from build123d import *

# Parameters (mm, degrees)
F1_DEPTH = 1.5875


with BuildPart() as f1:
    # F0 (on Front) → F1 (new body, symmetric)
    with BuildSketch(Plane.XZ):
        with BuildLine():
            Line((4.516544, 39.664961), (0, 39.664961))
            Line((0, 39.664961), (-4.516544, 39.664961))
            Line((-4.516544, 39.664961), (-8.198804, 45.188352))
            Line((-8.198804, 45.188352), (-8.198804, 39.664961))
            ThreePointArc((-8.198804, 39.664961), (-22.375505, 31.529893), (-36.552206, 39.664961))
            Line((-36.552206, 39.664961), (-63.432701, 39.664961))
            ThreePointArc((-63.432701, 39.664961), (-53.299794, 33.172534), (-54.963503, 21.253662))
            Line((-54.963503, 21.253662), (-38.393334, 21.253662))
            ThreePointArc((-38.393334, 21.253662), (-18.023802, 17.746605), (0, 7.629301))
            ThreePointArc((0, 7.629301), (18.023802, 17.746605), (38.393334, 21.253662))
            Line((38.393334, 21.253662), (54.963503, 21.253662))
            ThreePointArc((54.963503, 21.253662), (53.299794, 33.172534), (63.432701, 39.664961))
            Line((63.432701, 39.664961), (36.552206, 39.664961))
            ThreePointArc((36.552206, 39.664961), (22.375505, 31.529893), (8.198804, 39.664961))
            Line((8.198804, 39.664961), (8.198804, 45.188352))
            Line((8.198804, 45.188352), (4.516544, 39.664961))
        make_face()
    extrude(amount=F1_DEPTH, both=True)


solid = f1.part
Geometry: final body of the model. Coordinates: model frame, mm. A direction names the side the tool comes from. Round coordinates to 2 decimals unless told otherwise and drop trailing zeros. Order: outer loops, then holes, each group sorted by start corner. A loop starts at its lowest first (then second) coordinate and runs counter-clockwise, first axis right, second up. Notation, with made-up numbers: (6, 47.5) -> (20, 47.5) arc R21 ccw to (20, 67.5) -> close; hole circle Ø5 at (58.5, 53). An arc over 180 degrees is marked (long way). Put each result on its own line as item: value. Start each with the question number.
Q1. Line query: probe 1 along X at (y, z) = (0.25, 33.5); probe 2 along Z at (x, y) = (-39, -0.6); probe 3 along X at (y, z) = (-1.3, 41.5). Output: solid intervals per line, ascending.
Q2. Section D-D on x = -27.5. Return the cut outline in (y, z), and give its area (3 significant figures).
Q3. Section C-C on z = 36. Return the cut outline in (x, y).
Q4. Reachability of faces 1 (the flat face through (-47, 0, 21.254)), 2 (the flat face through (8.199, 0, 42)), 3 (the flat face through (0, 0, 39.665)), 4 (the flat face through (-8.199, 0, 42)) from +Z, -Z, +X, -X, +Y, -Y: full face, straight path, thin tool, end or side. Return the list, or none.
Q5. Pull-direction query (X, two-part tool) for faces 5 (the flat face through (-6.332, -0.022, 42.388)), 6 (the flat face through (6.383, -0.022, 42.465)), 7 (the cylindrical face through (-53.375, -0.022, 33.334)), 8 (the flat face through (-1, -1.588, 27)); classes: +X half, -X half, draft (parallel to the pull), parting line (faces both ways), or undercut.
Q6. Section B-B on y = -0.8. Return the cut outline in (x, z), and give its area (3 significant figures).
Q7. First-contact query: pin 1 (1.6 mm diameter, centred on x = 48.5, y = 0.5, fed in from +Z); pin 2 (1 mm diameter, centred on y = -1, z = 23, fed in from -X); pin 3 (1 mm diameter, centred on x = 44.5, y = -0.5, fed in from -Z). Flat tips, straight axial feed; report the tip coordinate or a pass-through.
Q8. Section A-A on z = 43. Return the cut outline in (x, y).
Ans:
1. probe 1: x = -53.46 to -30.17, -14.58 to 14.58, 30.17 to 53.46
1. probe 2: z = 21.25 to 39.66
1. probe 3: x = -8.2 to -5.74, 5.74 to 8.2
2. outline: (-1.59, 20.27) -> (1.59, 20.27) -> (1.59, 32.35) -> (-1.59, 32.35) -> close
2. area: 38.3 mm2
3. outline: (-55.17, -1.59) -> (-33.64, -1.59) -> (-33.64, 1.59) -> (-55.17, 1.59) -> close; (-11.11, -1.59) -> (11.11, -1.59) -> (11.11, 1.59) -> (-11.11, 1.59) -> close; (33.64, -1.59) -> (55.17, -1.59) -> (55.17, 1.59) -> (33.64, 1.59) -> close
4. face 1: -Z, -X, +Y, -Y
4. face 2: +Z, +X, +Y, -Y
4. face 3: +Z, +Y, -Y
4. face 4: +Z, -X, +Y, -Y
5. face 5: undercut
5. face 6: undercut
5. face 7: -X half
5. face 8: draft
6. outline: (-63.43, 39.66) arc R11.15 cw to (-54.96, 21.25) -> (-38.39, 21.25) arc R60.91 cw to (0, 7.63) arc R60.91 cw to (38.39, 21.25) -> (54.96, 21.25) arc R11.15 cw to (63.43, 39.66) -> (36.55, 39.66) arc R16.42 cw to (8.2, 39.66) -> (8.2, 45.19) -> (4.52, 39.66) -> (-4.52, 39.66) -> (-8.2, 45.19) -> (-8.2, 39.66) arc R16.42 cw to (-36.55, 39.66) -> close
6. area: 2,020 mm2
7. pin 1: stops at z = 39.66
7. pin 2: stops at x = -54.04
7. pin 3: stops at z = 21.25
8. outline: (-8.2, -1.59) -> (-6.74, -1.59) -> (-6.74, 1.59) -> (-8.2, 1.59) -> close; (6.74, -1.59) -> (8.2, -1.59) -> (8.2, 1.59) -> (6.74, 1.59) -> close
